Check sheet for the drawn part. Datum: minimum x, y, z corner. Units: mm. A direction names the side the tool comes from. Round coordinates to 2 decimals unless told otherwise and drop trailing zeros. Order: outer loops, then holes, each group sorted by start corner. A loop starts at its lowest first (then second) coordinate and runs counter-clockwise, first axis right, second up. Notation, with made-up numbers: M 89,-27.75 L 132,-27.75 A7 ccw 132,-20.75 Z; hole C 30,-33.75 d8. An arc over 180 degrees is marked long. Answer as a JSON object with one key per item and string values. Group by question number.
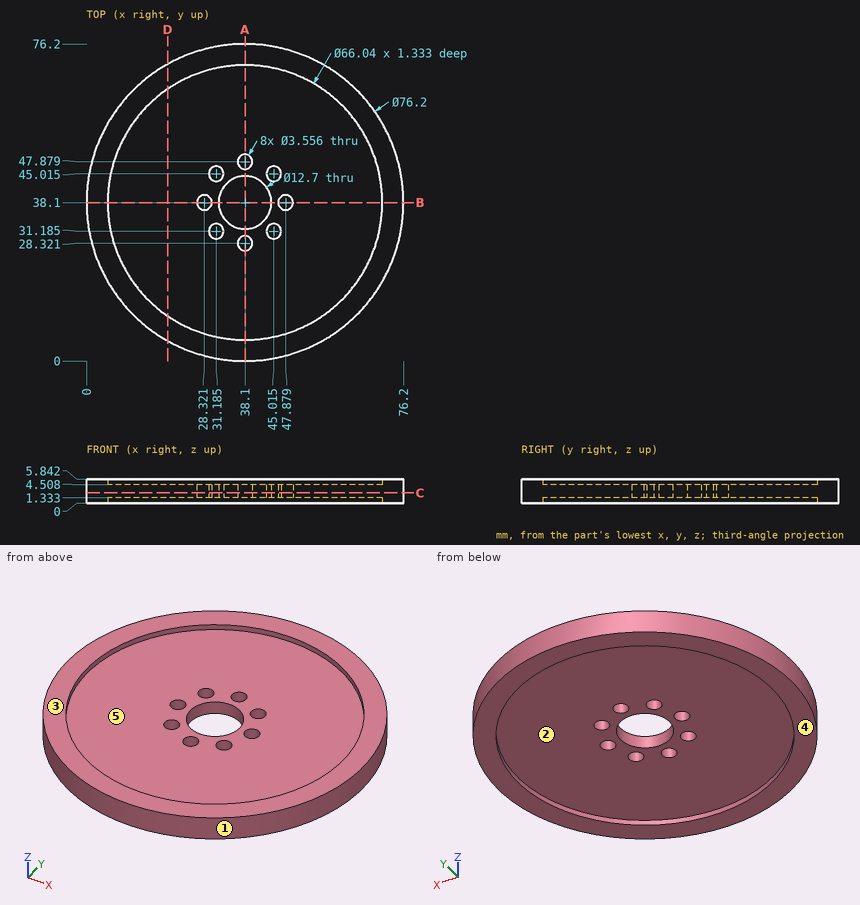
1) Thickness scan on line 1 along Y through (x, z) = (39.5, 2) (1 decimal); line 2 along Z through (x, y) = (43, 51.5); line 3 along Y through (x, z) = (63, 4.8) (1 decimal). Record the ranges inside material, lowest first. Write a range as [from, to].
2) Sectioned sample at C-C (z = 2.5). Count the separate pieces of the cut face and the enclosed holes in it, then the cut area to 3 significant figures.
3) Go/stop test with flat-tipped pins: P1, Ø2, axis at x = 31.19, y = 31.19, coming from the +Z side; P2, Ø4, axis at x = 38.1, y = 28.321, coming from the +Z side; P3, Ø14.5, axis at x = 38.1, y = 38.1, coming from the -Z side; P4, Ø8, axis at x = 63, y = 21.5, coming from the -Z side. Record where each tip stops, or that it passes through.
4) Release check for a two-part mould opening along Y. For the marked faces 1, 2 and 3 record: +Y half, -Y half, draft (parallel to the pull), parting line (faces both ways), or undercut.
5) Sectioned sample at A-A (x = 38.1). Record the boundary of the cut face in (y, z), then the cut area to 3 significant figures.
6) Sectioned sample at D-D (x = 19.5). Record the boundary of the cut face in (y, z).
7) Set-up check for the marked faces 4 and 5: record each of +Z, -Z, +X, -X, +Y, -Y from which the full face is reachable in a straight line by a thin tool's end or side.
Final values:
{
 "1": {"line 1": "y = [0, 27.2], [29.4, 31.9], [44.3, 46.8], [49, 76.2]", "line 2": "z = [1.33, 4.51]", "line 3": "y = [9.3, 16.4], [59.8, 66.9]"},
 "2": {"separate pieces": "1", "enclosed holes": "9", "area": "4,350 mm^2"},
 "3": {"P1": "passes through", "P2": "stops at z = 4.51", "P3": "stops at z = 1.33", "P4": "stops at z = 0"},
 "4": {"face 1": "parting line", "face 2": "undercut", "face 3": "draft"},
 "5": {"outline": "M 0,0 L 5.08,0 L 5.08,1.33 L 26.54,1.33 L 26.54,4.51 L 5.08,4.51 L 5.08,5.84 L 0,5.84 Z; M 30.1,1.33 L 31.75,1.33 L 31.75,4.51 L 30.1,4.51 Z; M 44.45,1.33 L 46.1,1.33 L 46.1,4.51 L 44.45,4.51 Z; M 49.66,1.33 L 71.12,1.33 L 71.12,0 L 76.2,0 L 76.2,5.84 L 71.12,5.84 L 71.12,4.51 L 49.66,4.51 Z", "area": "206 mm^2"},
 "6": {"outline": "M 4.85,0 L 10.82,0 L 10.82,1.33 L 65.38,1.33 L 65.38,0 L 71.35,0 L 71.35,5.84 L 65.38,5.84 L 65.38,4.51 L 10.82,4.51 L 10.82,5.84 L 4.85,5.84 Z"},
 "7": {"face 4": "-Z, +X, -X, +Y, -Y", "face 5": "+Z"}
}
